Check sheet for the modelled part. Datum: model origin and axes. Units: mm. Face numbers are marked on the shaded views. Give positions to 0.01 mm unless a question says otherwise; leave off trailing zeros. Write each loop counter-clockwise with the first axis right and the second up, starting at its lowest first coordinate (ties: lowest second). Pieces come first, ordered by that corner, then holes. Notation, with made-up numbers: M 6.5,67.5 L 10.5,67.5 A19 ccw 10.5,75.5 Z; hole C 80.5,24 d10. An arc over 180 degrees is marked long. Write item = value, one per line. Start each with the question number.
1) Sectioned sample at C-C, the plane y = 31.5. Record the cut outline in (x, z), then the cut area to 3 significant figures.
2) Draft check along X on the marked faces 1, 2 and 3. Enter one of: pulls with the +X half, pulls with the -X half, needs draft (parallel to the pull), parting line crosses it, or undercut.
3) Gauge pin test, flat end, axial feed: pin 1 (4 mm diameter, centred on x = 2.5, y = 26, fed in from -Z). Record the tip position at first contact, or that the pin passes through.
4) Sectioned sample at B-B, the plane z = 0. Record the cut outline in (x, y).
5) Sectioned sample at A-A, the plane x = 0. Record the cut outline in (y, z).
6) Scan lines: L1, parallel to Y at x = 0.75, z = 0.5; L2, parallel to Z at x = -1.5, y = 34; L3, parallel to Y at x = -1.25, z = -3. Record each from-to range of solid material in increasing order.
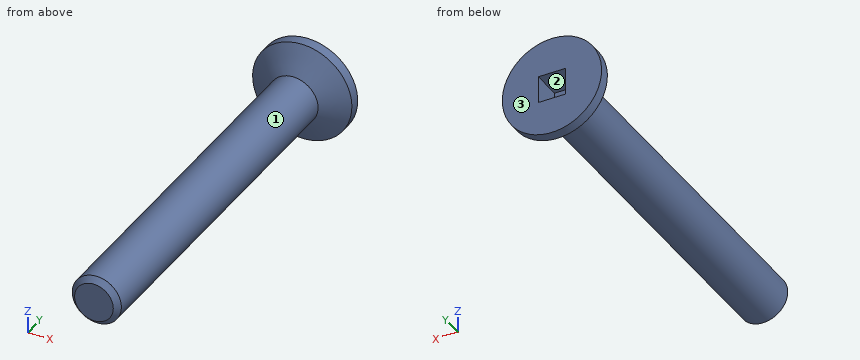
from build123d import *

# Parameters (mm, degrees)
SKETCH1_R           = 2.35
BOSS_EXTRUDE1_DEPTH = 37
CHAMFER1_SIZE       = 0.5
SKETCH3_W           = 2.6
SKETCH3_H           = 2.6
CUT_EXTRUDE1_DEPTH  = 2.8


with BuildPart() as part:
    # Sketch1 → Boss-Extrude1 (new body)
    with BuildSketch(Plane(origin=(0, 0, 0), x_dir=(1, 0, 0), z_dir=(0, 1, 0))):
        Circle(SKETCH1_R)
    extrude(amount=BOSS_EXTRUDE1_DEPTH)

    # Sketch2 → Revolve1 (revolve)
    with BuildSketch(Plane(origin=(0, 0, 0), x_dir=(0, 0, -1), z_dir=(1, 0, 0))):
        Polygon((0, 37), (-4.75, 37), (-4.75, 36), (0, 33), align=None)
    revolve(axis=Axis((0, 33, 0), (0, -1, 0)))

    # Chamfer1
    chamfer1_edges = [part.edges().sort_by_distance(p)[0] for p in [
        (-2.35, 0, 0),
    ]]
    chamfer(chamfer1_edges, length=CHAMFER1_SIZE)

    # Sketch3 → Cut-Extrude1 (cut)
    with BuildSketch(Plane(origin=(0, 37, 0), x_dir=(1, 0, 0), z_dir=(0, 1, 0))):
        Rectangle(SKETCH3_W, SKETCH3_H)
    extrude(amount=-CUT_EXTRUDE1_DEPTH, mode=Mode.SUBTRACT)


solid = part.part
Data:
q1.outline = C 0,0 d4.7
q1.area = 17.3 mm2
q2.face_1 = parting line crosses it
q2.face_2 = undercut
q2.face_3 = needs draft
q3.pin_1 = -2.3
q4.outline = M -4.75,36 L -2.35,34.48 L -2.35,0.5 L -1.85,0 L 1.85,0 L 2.35,0.5 L 2.35,34.48 L 4.75,36 L 4.75,37 L 1.3,37 L 1.3,34.2 L -1.3,34.2 L -1.3,37 L -4.75,37 Z
q5.outline = M 0,-1.85 L 0.5,-2.35 L 34.48,-2.35 L 36,-4.75 L 37,-4.75 L 37,-1.3 L 34.2,-1.3 L 34.2,1.3 L 37,1.3 L 37,4.75 L 36,4.75 L 34.48,2.35 L 0.5,2.35 L 0,1.85 Z
q6.L1 = 0 to 34.2
q6.L2 = -1.81 to 1.81
q6.L3 = 35.05 to 37
